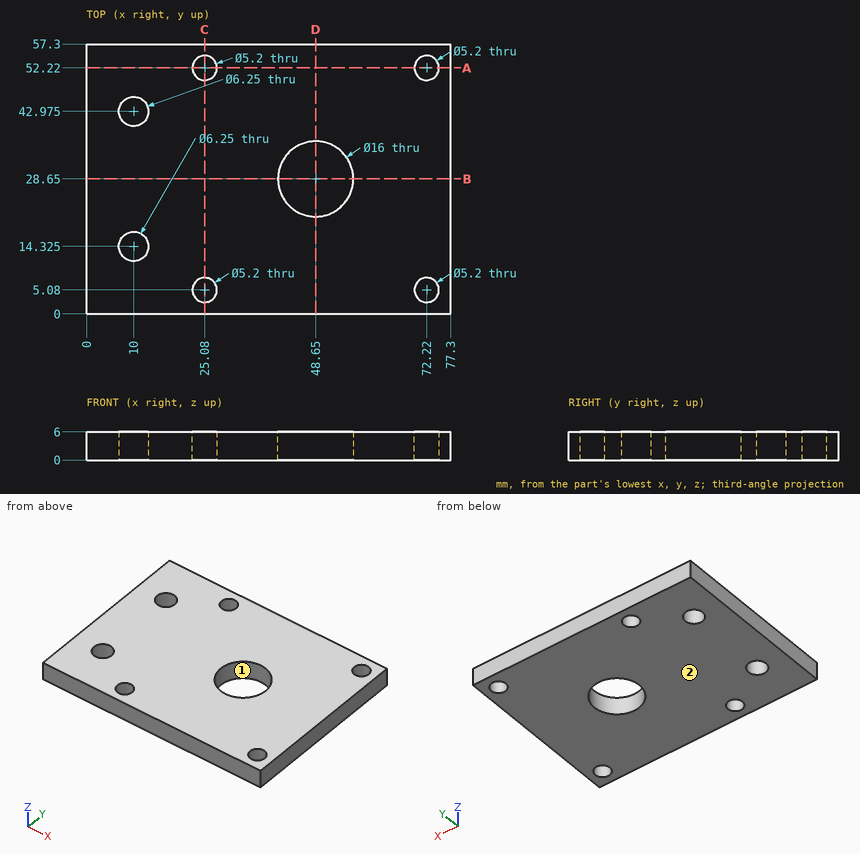
Could you check a few things on this drawing? It's one solid part, dimensions in mm from its lowest x, y, z. Coordinates: 2 decimals unless noted, no trailing zeros. Write each loop counter-clockwise with the first axis right and the second up, starting at its lowest first coordinate (ties: lowest second). Pieces come first, ordered by that corner, then holes. Notation, with made-up numbers: (-20, 86) - (-15, 86) arc R29 cw to (-15, 115) - close; hole circle Ø10 at (88, 6.5). An arc over 180 degrees is marked (long way). Return JSON: item names as keys, results as strings. Group by question number.
Item 1: Please list where these lines run through material, in increasing order: probe 1 along Y at (x, z) = (25.08, 4.85); probe 2 along Y at (x, z) = (10, 3.3); probe 3 along X at (y, z) = (51, 5.1).
Item 2: I'm going to push a flat-ended pin straight in: pin 1 Ø4 at (x, y) = (25.08, 5.08) entering from -Z (1 decimal). Where does the tip first touch, or does it pass through?
Item 3: If we section it at A-A (y = 52.22): Write out the boundary of the cut face in (x, z), then the cut area to 3 significant figures.
Item 4: If we section it at C-C (x = 25.08): Write out the boundary of the cut face in (y, z).
Item 5: If we section it at D-D (x = 48.65): Write out the boundary of the cut face in (y, z).
Item 6: We'd pull the mould along Y, two halves only. Please class the marked faces 1 and 2: pulls with the +Y half, pulls with the -Y half, needs draft (parallel to the pull), parting line crosses it, or undercut.
Item 7: If we section it at B-B (y = 28.65): Write out the boundary of the cut face in (x, z), then the cut area to 3 significant figures.
Return value:
{
 "1": {"probe 1": "y = 0 to 2.48, 7.68 to 49.62, 54.82 to 57.3", "probe 2": "y = 0 to 11.2, 17.45 to 39.85, 46.1 to 57.3", "probe 3": "x = 0 to 22.78, 27.38 to 69.92, 74.52 to 77.3"},
 "2": {"pin 1": "passes through"},
 "3": {"outline": "(0, 0) - (22.48, 0) - (22.48, 6) - (0, 6) - close; (27.68, 0) - (69.62, 0) - (69.62, 6) - (27.68, 6) - close; (74.82, 0) - (77.3, 0) - (77.3, 6) - (74.82, 6) - close", "area": "401 mm^2"},
 "4": {"outline": "(0, 0) - (2.48, 0) - (2.48, 6) - (0, 6) - close; (7.68, 0) - (49.62, 0) - (49.62, 6) - (7.68, 6) - close; (54.82, 0) - (57.3, 0) - (57.3, 6) - (54.82, 6) - close"},
 "5": {"outline": "(0, 0) - (20.65, 0) - (20.65, 6) - (0, 6) - close; (36.65, 0) - (57.3, 0) - (57.3, 6) - (36.65, 6) - close"},
 "6": {"face 1": "undercut", "face 2": "needs draft"},
 "7": {"outline": "(0, 0) - (40.65, 0) - (40.65, 6) - (0, 6) - close; (56.65, 0) - (77.3, 0) - (77.3, 6) - (56.65, 6) - close", "area": "368 mm^2"}
}
